Read the model definition and answer for the solid it produces. Units are mm, in the model's axes. A direction names the side the tool comes from. Coordinates: 2 decimals unless noted, no trailing zeros. Write each loop counter-clockwise with the first axis right and the second up, starting at its lowest first coordinate (ties: lowest second). Pieces come first, ordered by that corner, then holes. Notation, with made-up numbers: M 33.25,22 L 65.25,22 A12 cw 65.25,44 Z; hole C 71,-17 d9. An arc over 180 degrees is marked long. Use a Markdown table: item, result. Add a question column.
Autodesk Fusion 360 part; units mm, degrees
sketch "Sketch1" plane through (0, 0, 0) normal (0, 0, 1) x (1, 0, 0)
  line L0 (65.5, -65.5) -> (-65.5, -65.5) construction
  line L1 (-65.5, -65.5) -> (-65.5, 65.5) construction
  line L2 (-65.5, 65.5) -> (65.5, 65.5) construction
  line L3 (65.5, 65.5) -> (65.5, -65.5) construction
  line L4 (65.5, -65.5) -> (-65.5, 65.5) construction
  line L5 (-65.5, -65.5) -> (65.5, 65.5) construction
  line L6 (0, 50) -> (0, -50) construction
  line L7 (-50, 0) -> (50, 0) construction
  line L8 (-60, 60.5) -> (5, 60.5)
  line L9 (5, 60.5) -> (5, -60.5)
  line L10 (5, -60.5) -> (-60, -60.5)
  line L11 (-60, -60.5) -> (-60, 60.5)
  circle A0 centre (-50, 0) radius 2.5
  circle A1 centre (0, 50) radius 2.5
  circle A2 centre (0, -50) radius 2.5
  line L12 (-54.4646, 20.8308) -> (-5.4646, 20.8308) construction
  line L13 (-5.4646, 20.8308) -> (-5.4646, -37.1692) construction
  line L14 (-5.4646, -37.1692) -> (-54.4646, -37.1692) construction
  line L15 (-54.4646, -37.1692) -> (-54.4646, 20.8308) construction
  circle A3 centre (-54.4646, 20.8308) radius 1.15
  circle A4 centre (-54.4646, 20.8308) radius 2.65
  circle A5 centre (-5.4646, 20.8308) radius 1.15
  circle A6 centre (-5.4646, 20.8308) radius 2.65
  circle A7 centre (-54.4646, -37.1692) radius 1.15
  circle A8 centre (-54.4646, -37.1692) radius 2.65
  circle A9 centre (-5.4646, -37.1692) radius 1.15
  circle A10 centre (-5.4646, -37.1692) radius 2.65
  line L16 (-45, 2.5) -> (-13.4646, 2.5)
  line L17 (-13.4646, 2.5) -> (-13.4646, 55.5)
  line L18 (-13.4646, 55.5) -> (-45, 55.5)
  line L19 (-45, 55.5) -> (-45, 2.5)
  line L20 (-45, -2.5) -> (-13.4646, -2.5)
  line L21 (-13.4646, -2.5) -> (-13.4646, -55.5)
  line L22 (-13.4646, -55.5) -> (-45, -55.5)
  line L23 (-45, -55.5) -> (-45, -2.5)
  point P0 (5, 0)
  dimension "d4" = 131
  dimension "d5" = 131
  dimension "d6" = 100
  dimension "d7" = 100
  dimension "d8" = 5
  dimension "d9" = 5
  dimension "d10" = 5
  dimension "d14" = 5
  dimension "d15" = 10
  dimension "d16" = 49
  dimension "d17" = 58
  dimension "d18" = 2.3
  dimension "d19" = 1.5
  dimension "d22" = 49
  dimension "d23" = -58
  dimension "d32" = 5
  dimension "d33" = 5
  dimension "d35" = 8
  dimension "d36" = 2.5
  dimension "d37" = 2.5
  dimension "d38" = 5
  dimension "d39" = 5
  dimension "d40" = 8
  dimension "d41" = 5
  dimension "d42" = 5
extrude "Extrude1" add sketch "Sketch1" along normal blind 2 contours L8 L9 L10 L11 | A3 | A4 | A5 | A6 | A7 | A8 | A9 | A10
extrude "Extrude2" add sketch "Sketch1" along normal blind 6.5 contours A4 | A6 | A8 | A10
draft "Draft1" angle 30 neutral plane through (0, 0, 6.5) pull (0, 0, 1) 4 faces at (-51.8278, -36.9053, 3.5) (-51.8278, 21.0947, 3.5) (-2.8278, 21.0947, 3.5) (-2.8278, -36.9053, 3.5)
fillet "Fillet1" radius 5 12 edges at (-60, -60.5, 1) (5, -60.5, 1) (5, 60.5, 1) (-60, 60.5, 1) (-45, 55.5, 1) (-13.4646, 55.5, 1) (-13.4646, 2.5, 1) (-45, 2.5, 1) (-45, -2.5, 1) (-13.4646, -2.5, 1) (-13.4646, -55.5, 1) (-45, -55.5, 1)
Item 1: Find section C-C on x = -15. Give the vertices of the cut face in (y, z).
Item 2: Each of these flat-tipped pins is pushed along its axis until it touches: pin 1 (0.7 mm diameter, centred on x = -6, y = -37.5, fed in from +Z); pin 2 (2.5 mm diameter, centred on x = -54.46, y = 20.83, fed in from -Z). Where does it stop, or does it pass through?
Item 3: Consider probe 1 along Y at (x, z) = (-22, 1); probe 2 along Y at (x, z) = (0, 1); probe 3 along X at (y, z) = (-19, 1.25). Determine where each line is inside the solid, lowest interval first.
Item 4: Find section B-B on z = 5.25. Give the vertices of the cut face in (x, y).
Item 5: Find section D-D on y = 0. Give the vertices of the cut face in (x, z), then the cut area to 3 significant figures.
Item 6: Determine the mould class of faces 4 (the cylindrical face through (-14.89, -4.004, 1.014)), 5 (the flat face through (-53, 20, 6.5)), 6 (the cylindrical face through (3.57, 59, 1.01)), 7 (the cylindrical face through (-58.57, -59, 1.01)) for opening direction X: pulls with the +X half, pulls with the -X half, needs draft (parallel to the pull), parting line crosses it, or undercut.
Item 7: For faces 1 (the cylindrical face through (-58.5, 59.07, 1.01)), 2 (the cylindrical face through (-14.968, -54.074, 1.014)), 3 (the cylindrical face through (-5.714, -36.047, 4.219)), determine the directions among +Z, -Z, +X, -X, +Y, -Y from which every point of the face is accessible in a straight line to the end or side of a thin tool.
Item 8: Find section A-A on y = -16.5. Give the vertices of the cut face in (x, z).
Geometry says:
| question | item | result |
|---|---|---|
| 1 | outline | M -60.5,0 L -54.11,0 L -54.11,2 L -60.5,2 Z; M -3.89,0 L 3.89,0 L 3.89,2 L -3.89,2 Z; M 54.11,0 L 60.5,0 L 60.5,2 L 54.11,2 Z |
| 2 | pin 1 | stops at z = 2 |
| 2 | pin 2 | stops at z = 0 |
| 3 | probe 1 | y = -60.5 to -55.5, -2.5 to 2.5, 55.5 to 60.5 |
| 3 | probe 2 | y = -60.5 to -52.5, -47.5 to 47.5, 52.5 to 60.5 |
| 3 | probe 3 | x = -60 to -45, -13.46 to 5 |
| 4 | outline | C -54.46,-37.17 d6.74; C -54.46,20.83 d6.74; C -5.46,-37.17 d6.74; C -5.46,20.83 d6.74; hole C -54.46,-37.17 d2.3; hole C -54.46,20.83 d2.3; hole C -5.46,-37.17 d2.3; hole C -5.46,20.83 d2.3 |
| 5 | outline | M -60,0 L -52.5,0 L -52.5,2 L -60,2 Z; M -47.5,0 L 5,0 L 5,2 L -47.5,2 Z |
| 5 | area | 120 mm2 |
| 6 | face 4 | undercut |
| 6 | face 5 | needs draft |
| 6 | face 6 | pulls with the +X half |
| 6 | face 7 | pulls with the -X half |
| 7 | face 1 | +Z, -Z, -X, +Y |
| 7 | face 2 | +Z, -Z |
| 7 | face 3 | +Z |
| 8 | outline | M -60,0 L -45,0 L -45,2 L -60,2 Z; M -13.46,0 L 5,0 L 5,2 L -13.46,2 Z |
